Build history of the part. All positions in model axes, mm. Give positions to 0.01 mm unless a question says otherwise; leave off trailing zeros. Order: outer loops, then holes, each group sorted by start corner. A loop starts at its lowest first (then second) coordinate and runs counter-clockwise, first axis right, second up. Notation, with made-up numbers: (-26.5, 17) - (23.5, 17) arc R20 cw to (23.5, 38) - close; hole circle Ø4 at (11, -27). An arc over 180 degrees is marked (long way). Use a Markdown table: item, result.
from build123d import *

# Parameters (mm, degrees)
CONG_1_R                     = 2
BOSS_EXTRU_1_DEPTH           = 40
ESQUISSE3_R                  = 3
ENL_V_MAT_EXTRU_1_DEPTH      = 22.074664225
ENL_V_MAT_EXTRU_1_DEPTH_BACK = 22.074664225


with BuildPart() as part:
    # Esquisse1 → Révolution1 (revolve)
    with BuildSketch(Plane.XY):
        with BuildLine():
            Line((-2.05, 0), (-2.05, 40))
            Line((-2.05, 40), (-22.05, 40))
            ThreePointArc((-22.05, 40), (-17.818604845, 20), (-22.05, 0))
            Line((-22.05, 0), (-2.05, 0))
        make_face()
    revolve(axis=Axis((0, 0, 0), (0, 1, 0)))

    # Congé1
    cong_1_edges = [part.edges().sort_by_distance(p)[0] for p in [
        (22.05, 40, 0),
        (22.05, 0, 0),
    ]]
    fillet(cong_1_edges, radius=CONG_1_R)

    # Esquisse2 → Boss.-Extru.1 (add)
    with BuildSketch(Plane(origin=(0, 40, 0), x_dir=(1, 0, 0), z_dir=(0, 1, 0))):
        with BuildLine():
            Line((-1.5, 1.397318861), (1.5, 1.397318861))
            ThreePointArc((1.5, 1.397318861), (0, 2.05), (-1.5, 1.397318861))
        make_face()
    extrude(amount=-BOSS_EXTRU_1_DEPTH)

    # Esquisse3 → Enlèv. mat.-Extru.1 (cut, two sides)
    with BuildSketch(Plane.XY) as enl_v_mat_extru_1_sk:
        with Locations((-10.821847214, 20)):
            Circle(ESQUISSE3_R)
    extrude(amount=ENL_V_MAT_EXTRU_1_DEPTH, mode=Mode.SUBTRACT)
    extrude(enl_v_mat_extru_1_sk.sketch, amount=-ENL_V_MAT_EXTRU_1_DEPTH_BACK, mode=Mode.SUBTRACT)


solid = part.part
1) Two-plate mould, pull along Z, no slides. Class faces 1 (the flat face through (4, 40, 0)), 2 (the flat face through (0, 20, -1.397)): +Z half, -Z half, draft (parallel to the pull), parting line (faces both ways), or undercut.
Computed:
| item | result |
|---|---|
| face 1 | draft |
| face 2 | undercut |
2) Slice it at C-C (y = 33). Write the cut outline in (x, z).
Computed:
| item | result |
|---|---|
| outline | circle Ø39.12 at (0, 0); hole (-1.5, -1.4) - (1.5, -1.4) arc R2.05 ccw (long way) to start |
3) Wall check: line 1 (X direction, y = 20, z = 0); line 2 (X direction, y = 17.5, z = -4.5); line 3 (Z direction, x = 0, y = 15). Give the ranges that are in metal, low to high. Write a range as from..to.
Computed:
| item | result |
|---|---|
| line 1 | x = -17.82..-13.82, -7.82..-2.05, 2.05..17.82 |
| line 2 | x = -17.31..-12.48, -9.16..17.31 |
| line 3 | z = -18.07..-1.4, 2.05..18.07 |
4) Slice it at B-B (y = 22). Write the cut outline in (x, z).
Computed:
| item | result |
|---|---|
| outline | (-13.06, -12.18) - (-13.06, 12.18) arc R17.86 ccw to start; (-8.59, -15.66) arc R17.86 ccw (long way) to (-8.59, 15.66) - close; hole (-1.5, -1.4) - (1.5, -1.4) arc R2.05 ccw (long way) to start |
5) Pin check, flat tips, straight feed: P1, Ø6, axis at x = 8, y = 8.5, coming from the +Z side; P2, Ø2, axis at x = -7, y = 9.5, coming from the -Z side; P3, Ø5, axis at y = 25, z = -14, coming from the +X side. Stop position of each tip, or through.
Computed:
| item | result |
|---|---|
| P1 | stops at z = 18.84 |
| P2 | stops at z = -18.05 |
| P3 | stops at x = 13.97 |
6) Slice it at A-A (z = 0). State how many separate pieces and enclosed holes the cut face has, and give its area (3 significant figures).
Computed:
| item | result |
|---|---|
| separate pieces | 2 |
| enclosed holes | 1 |
| area | 1,340 mm² |
